Input: part model. Units: mm. Frame: model coordinates. Face numbers are marked on the shaded views. A direction names the side the tool comes from. Round coordinates to 2 decimals unless told otherwise and drop trailing zeros. Loops run counter-clockwise (first coordinate to the right, second up) from the corner with the lowest first, then second, coordinate; pieces in that order, holes last. Notation, with made-up numbers: (87.25, 64.25) - (93.25, 64.25) arc R23 cw to (93.25, 94.25) - close; hole circle Ø6 at (7, 32.5). An arc over 180 degrees is marked (long way). One line per question, with ' | ' between items. Start each with the question number.
from build123d import *

# Parameters (mm, degrees)
SKETCH1_R           = 52.5
BOSS_EXTRUDE1_DEPTH = 13
SKETCH2_R           = 17.5
BOSS_EXTRUDE2_DEPTH = 7
SKETCH3_R           = 52.5
SKETCH3_R_2         = 25
CUT_EXTRUDE1_DEPTH  = 8
SKETCH4_R           = 7.5
CUT_EXTRUDE2_DEPTH  = 77.892782496
SKETCH5_R           = 10.5
CUT_EXTRUDE3_DEPTH  = 5
SKETCH6_R           = 3.5
CUT_EXTRUDE4_DEPTH  = 2.5


with BuildPart() as part:
    # Sketch1 → Boss-Extrude1 (new body)
    with BuildSketch(Plane.XY):
        with Locations(Location((0, 0, 0), (0, 0, 180))):
            Circle(SKETCH1_R)
    extrude(amount=BOSS_EXTRUDE1_DEPTH)

    # Sketch2 → Boss-Extrude2 (add)
    with BuildSketch(Plane(origin=(0, 0, 0), x_dir=(-1, 0, 0), z_dir=(0, 0, -1))):
        Circle(SKETCH2_R)
    extrude(amount=BOSS_EXTRUDE2_DEPTH)

    # Sketch3 → Cut-Extrude1 (cut)
    with BuildSketch(Plane(origin=(0, 0, 0), x_dir=(-1, 0, 0), z_dir=(0, 0, -1))):
        Circle(SKETCH3_R)
        Circle(SKETCH3_R_2, mode=Mode.SUBTRACT)
    extrude(amount=-CUT_EXTRUDE1_DEPTH, mode=Mode.SUBTRACT)

    # Sketch4 → Cut-Extrude2 (cut, through all)
    with BuildSketch(Plane(origin=(0, 0, -7), x_dir=(-1, 0, 0), z_dir=(0, 0, -1))):
        Circle(SKETCH4_R)
    extrude(amount=-CUT_EXTRUDE2_DEPTH, mode=Mode.SUBTRACT)

    # Sketch5 → Cut-Extrude3 (cut)
    with BuildSketch(Plane.XY.offset(13)):
        Circle(SKETCH5_R)
    extrude(amount=-CUT_EXTRUDE3_DEPTH, mode=Mode.SUBTRACT)

    # Sketch6 → Cut-Extrude4 (cut)
    with BuildSketch(Plane(origin=(0, 0, 13), x_dir=(-1, 0, 0), z_dir=(0, 0, -1))):
        with Locations((0, 44)):
            Circle(SKETCH6_R)
        with Locations((38.105117767, 22)):
            Circle(SKETCH6_R)
        with Locations((38.105117767, -22)):
            Circle(SKETCH6_R)
        with Locations((0, -44)):
            Circle(SKETCH6_R)
        with Locations((-38.105117767, -22)):
            Circle(SKETCH6_R)
        with Locations((-38.105117767, 22)):
            Circle(SKETCH6_R)
    extrude(amount=CUT_EXTRUDE4_DEPTH, mode=Mode.SUBTRACT)


solid = part.part
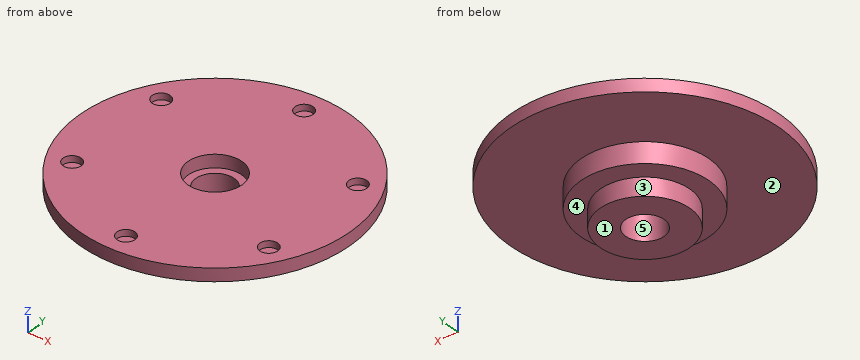
(1) Pin query (flat end, axial travel): P1, Ø2, axis at x = 39.5, y = -23, coming from the +Z side; P2, Ø5.5, axis at x = -38.11, y = -22, coming from the -Z side; P3, Ø8, axis at y = 35, z = 6, coming from the +X side; P4, Ø12, axis at x = 0, y = 0, coming from the -Z side. Return the tip coordinate at first contact, or that it passes through.
(2) Section B-B, the plane y = 44. Output: boundary loops of the cut face in (x, z).
(3) Line query: line 1 along Y through (x, z) = (0, 12); line 2 along Z through (x, y) = (-10, -36); line 3 along Z through (x, y) = (-7, -22). Output: solid intervals per line, ascending. Write a range as from..to.
(4) Section D-D, the plane z = -3.5. Output: boundary loops of the cut face in (x, y).
(5) Pull-direction query (Y, two-part tool) for the marked faces 3, 4 and 5; classes: released by +Y, released by -Y, zero draft, split by the parting line, or undercut.
(6) Section A-A, the plane x = 0. Output: boundary loops of the cut face in (y, z).
(7) Section C-C, the plane y = 0. Output: boundary loops of the cut face in (x, z).
(8) Reachability of the marked faces 1 and 2 from +Z, -Z, +X, -X, +Y, -Y: full face, straight path, thin tool, end or side. Return the list, or none.
Derived:
1) P1: stops at z = 10.5 | P2: stops at z = 8 | P3: stops at x = 41.97 | P4: passes through
2) outline: (-28.64, 8) - (28.64, 8) - (28.64, 13) - (3.5, 13) - (3.5, 10.5) - (-3.5, 10.5) - (-3.5, 13) - (-28.64, 13) - close
3) line 1: y = -52.5..-47.5, -40.5..-10.5, 10.5..40.5, 47.5..52.5 | line 2: z = 8..13 | line 3: z = 0..13
4) outline: circle Ø35 at (0, 0); hole circle Ø15 at (0, 0)
5) face 3: split by the parting line | face 4: zero draft | face 5: undercut
6) outline: (-52.5, 8) - (-25, 8) - (-25, 0) - (-17.5, 0) - (-17.5, -7) - (-7.5, -7) - (-7.5, 8) - (-10.5, 8) - (-10.5, 13) - (-40.5, 13) - (-40.5, 10.5) - (-47.5, 10.5) - (-47.5, 13) - (-52.5, 13) - close; (7.5, -7) - (17.5, -7) - (17.5, 0) - (25, 0) - (25, 8) - (52.5, 8) - (52.5, 13) - (47.5, 13) - (47.5, 10.5) - (40.5, 10.5) - (40.5, 13) - (10.5, 13) - (10.5, 8) - (7.5, 8) - close
7) outline: (-52.5, 8) - (-25, 8) - (-25, 0) - (-17.5, 0) - (-17.5, -7) - (-7.5, -7) - (-7.5, 8) - (-10.5, 8) - (-10.5, 13) - (-52.5, 13) - close; (7.5, -7) - (17.5, -7) - (17.5, 0) - (25, 0) - (25, 8) - (52.5, 8) - (52.5, 13) - (10.5, 13) - (10.5, 8) - (7.5, 8) - close
8) face 1: -Z, +X, -X, +Y, -Y | face 2: -Z
